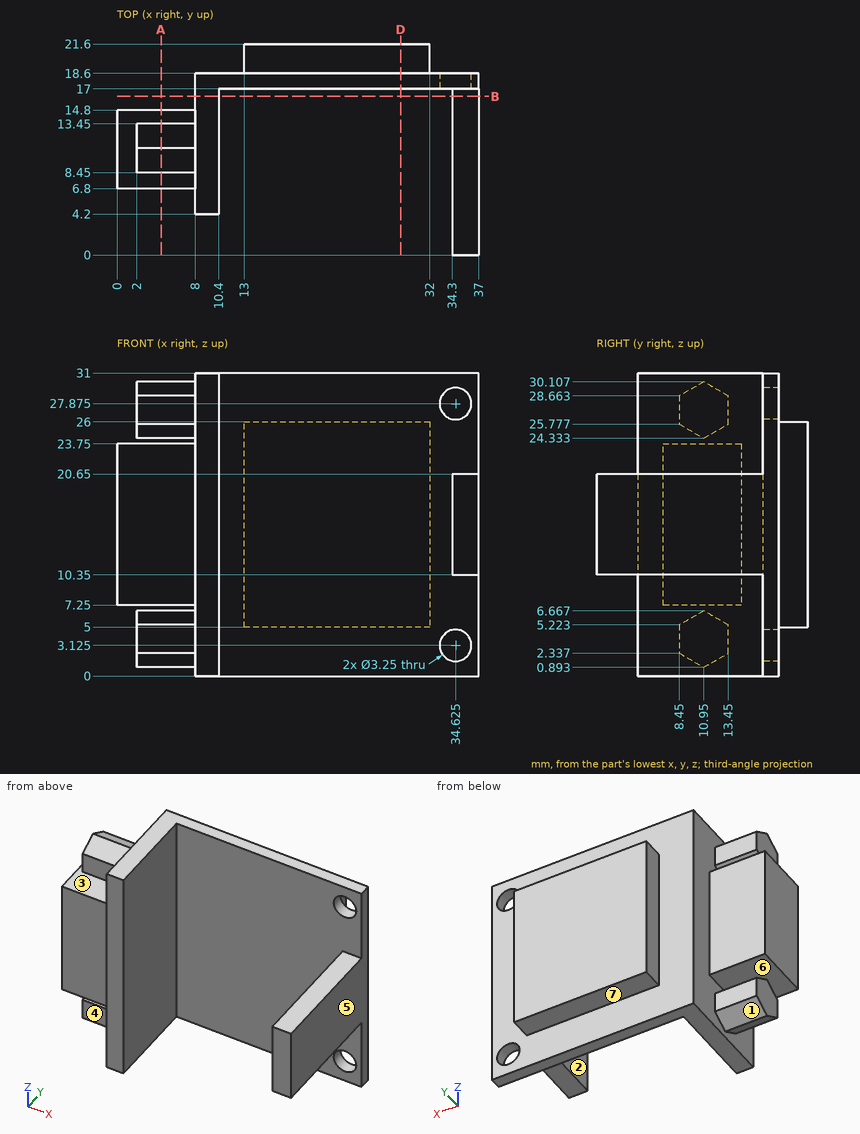
Source: three-view drawing plus pictorial views. Frame: mm from the lowest corner of the part. A direction names the side the tool comes from. Round coordinates to 2 decimals unless told otherwise and drop trailing zeros. Loops run counter-clockwise (first coordinate to the right, second up) from the corner with the lowest first, then second, coordinate; pieces in that order, holes last.
Q1. Material intervals for L1, parallel to X at y = 15.75, z = 11.5; L2, parallel to X at y = 10.75, z = 12; L3, parallel to Y at x = 6.5, z = 22.5, sorted ascending.
Q2. Pull-direction query (Z, two-part tool) for the marked faces 5, 6 and 7; classes: released by +Z, released by -Z, zero draft, split by the parting line, or undercut.
Q3. Section B-B on y = 16.25. Return loops of the section in (x, z).
Q4. Access query for the marked faces 1, 2, 3 and 4. Directions: +Z, -Z, +X, -X, +Y, -Y. A direction counts if a zero-diameter tool reaches every point of the face in a straight line with its end or side. Return the directions, or none.
Q5. Section D-D on x = 29. Return loops of the section in (y, z).
Q6. Section A-A on x = 4.5. Return loops of the section in (y, z), plus the area to 3 significant figures.
Q7. Pin query (flat end, axial travel): P1, Ø6.5, axis at x = 3, z = 19.5, coming from the +Y side; P2, Ø5, axis at x = 34.625, z = 3.125, coming from the -Y side; P3, Ø5, axis at x = 4, y = 18, coming from the +Z side; P4, Ø2.5, axis at x = 6, z = 3, coming from the -Y side. Return the tip coordinate at first contact, or that it passes through.
Evaluation:
1. L1: x = 8 to 10.4, 34.3 to 37
1. L2: x = 0 to 10.4, 34.3 to 37
1. L3: y = 6.8 to 14.8
2. face 5: zero draft
2. face 6: undercut
2. face 7: released by -Z
3. outline: (8, 0) - (10.4, 0) - (10.4, 31) - (8, 31) - close; (34.3, 10.35) - (37, 10.35) - (37, 20.65) - (34.3, 20.65) - close
4. face 1: -Z, -X, +Y
4. face 2: +Z, -Z, -Y
4. face 3: -X, +Y, -Y
4. face 4: -Z, -X, -Y
5. outline: (17, 0) - (18.6, 0) - (18.6, 5) - (21.6, 5) - (21.6, 26) - (18.6, 26) - (18.6, 31) - (17, 31) - close
6. outline: (6.8, 7.25) - (14.8, 7.25) - (14.8, 23.75) - (6.8, 23.75) - close; (8.45, 2.34) - (10.95, 0.89) - (13.45, 2.34) - (13.45, 5.22) - (10.95, 6.67) - (8.45, 5.22) - close; (8.45, 25.78) - (10.95, 24.33) - (13.45, 25.78) - (13.45, 28.66) - (10.95, 30.11) - (8.45, 28.66) - close
6. area: 175 mm2
7. P1: stops at y = 14.8
7. P2: stops at y = 17
7. P3: passes through
7. P4: stops at y = 8.45
